```python
from build123d import *

# Parameters (mm, degrees)
F1_DEPTH = 50
F2_W     = 2.5
F2_H     = 40
F2_W_2   = 50
F2_W_3   = 9
F2_W_4   = 21.211368
F3_DEPTH = 5
F4_W     = 40
F4_H     = 40
F5_DEPTH = 350
F6_W     = 9
F6_H     = 40
F6_W_2   = 2.5
F7_DEPTH = 25


with BuildPart() as f1:
    # F0 (on Front) → F1 (new body)
    with BuildSketch(Plane.XZ):
        Polygon((97.859602, 45), (-152.140398, 45), (-152.140398, -5), (97.859602, -5), (97.859602, 0), align=None)
        Polygon((-147.140398, 40), (-145.640398, 40), (-125.92903, 0), (-147.140398, 0), align=None, mode=Mode.SUBTRACT)
        Polygon((-90.06627, 40), (-111.354901, 0), (-120.354901, 0), (-140.06627, 40), align=None, mode=Mode.SUBTRACT)
        Polygon((-55.690862, 0), (-105.690862, 0), (-84.402231, 40), (-75.402231, 40), align=None, mode=Mode.SUBTRACT)
        Polygon((-50.116734, 0), (-69.828102, 40), (-19.828102, 40), (-41.116734, 0), align=None, mode=Mode.SUBTRACT)
        Polygon((-14.164063, 40), (-5.164063, 40), (14.547306, 0), (-35.452694, 0), align=None, mode=Mode.SUBTRACT)
        Polygon((20.121434, 0), (0.410065, 40), (50.410065, 40), (29.121434, 0), align=None, mode=Mode.SUBTRACT)
        Polygon((65.074105, 40), (84.785473, 0), (34.785473, 0), (56.074105, 40), align=None, mode=Mode.SUBTRACT)
        Polygon((92.859602, 40), (92.859602, 0), (90.359602, 0), (70.648233, 40), align=None, mode=Mode.SUBTRACT)
    extrude(amount=F1_DEPTH)

    # F2 (on face) → F3 (cut)
    with BuildSketch(Plane(origin=(0, 0, -5), x_dir=(1, 0, 0), z_dir=(0, 0, -1))):
        with Locations((91.609602, 25)):
            Rectangle(F2_W, F2_H)
        with Locations((59.785473, 25)):
            Rectangle(F2_W_2, F2_H)
        with Locations((-10.452694, 25)):
            Rectangle(F2_W_2, F2_H)
        with Locations((24.621434, 25)):
            Rectangle(F2_W_3, F2_H)
        with Locations((-80.690862, 25)):
            Rectangle(F2_W_2, F2_H)
        with Locations((-45.616734, 25)):
            Rectangle(F2_W_3, F2_H)
        with Locations((-136.534714, 25)):
            Rectangle(F2_W_4, F2_H)
        with Locations((-115.854901, 25)):
            Rectangle(F2_W_3, F2_H)
    extrude(amount=-F3_DEPTH, mode=Mode.SUBTRACT)

    # F4 (on face) → F5 (cut)
    with BuildSketch(Plane.YZ.offset(97.859602)):
        with Locations((-25, 20)):
            Rectangle(F4_W, F4_H)
    extrude(amount=-F5_DEPTH, mode=Mode.SUBTRACT)

    # F6 (on face) → F7 (cut)
    with BuildSketch(Plane(origin=(0, 0, 40), x_dir=(1, 0, 0), z_dir=(0, 0, -1))):
        Polygon((-145.640398, 5), (-140.06627, 5), (-125.92903, 5), (-125.92903, 45), (-140.06627, 45), (-145.640398, 45), (-147.140398, 45), (-147.140398, 5), align=None)
        with Locations((-115.854901, 25)):
            Rectangle(F6_W, F6_H)
        Polygon((-5.164063, 5), (0.410065, 5), (14.547306, 5), (14.547306, 45), (0.410065, 45), (-5.164063, 45), (-14.164063, 45), (-19.828102, 45), (-35.452694, 45), (-35.452694, 5), (-19.828102, 5), (-14.164063, 5), align=None)
        Polygon((-75.402231, 5), (-69.828102, 5), (-55.690862, 5), (-55.690862, 45), (-69.828102, 45), (-75.402231, 45), (-84.402231, 45), (-90.06627, 45), (-105.690862, 45), (-105.690862, 5), (-90.06627, 5), (-84.402231, 5), align=None)
        with Locations((-45.616734, 25)):
            Rectangle(F6_W, F6_H)
        with Locations((24.621434, 25)):
            Rectangle(F6_W, F6_H)
        Polygon((65.074105, 5), (70.648233, 5), (84.785473, 5), (84.785473, 45), (70.648233, 45), (65.074105, 45), (56.074105, 45), (50.410065, 45), (34.785473, 45), (34.785473, 5), (50.410065, 5), (56.074105, 5), align=None)
        with Locations((91.609602, 25)):
            Rectangle(F6_W_2, F6_H)
    extrude(amount=-F7_DEPTH, mode=Mode.SUBTRACT)


solid = f1.part
```
Work out the finished part from the listing and answer in its coordinate system (mm). A direction names the side the tool comes from. Give positions to 0.01 mm unless a question says otherwise; leave off trailing zeros. Loops run counter-clockwise (first coordinate to the right, second up) from the corner with the lowest first, then second, coordinate; pieces in that order, holes last. Notation, with made-up numbers: M 85,-22.5 L 91,-22.5 A21 cw 91,1.5 Z; hole C 70,82.5 d4. An arc over 180 degrees is marked long. One line per item, written item: value. Start each with the question number.
1. Find section B-B (x = 38.5). Give the vertices of the cut face in (y, z).
2. Find the intervals of material crossed by probe 1 along Y at (x, z) = (42.5, 23.5); probe 2 along Z at (x, y) = (-36, -20); probe 3 along Z at (x, y) = (11, -3), in increasing order.
3. Find section A-A (x = -11.5). Give the vertices of the cut face in (y, z).
4. Each of these flat-tipped pins is pushed along its axis until it touches: P1, Ø8, axis at x = -132, z = 13, coming from the +Y side; P2, Ø1.5, axis at y = -37.5, z = 38.5, coming from the -X side. Where does it stop, or does it pass through?
5. Which of the six approach directions +Z, -Z, +X, -X, +Y, -Y give full straight-line access (tool end or side, diameter ignored) to faces 1 (the face through (-111.355, -25, 42)), 2 (the face through (-24.957, -47.465, 19.72)), 3 (the face through (-123, -25, 0))?
6. Find section C-C (y = -25.5). State how many separate pieces and enclosed holes the cut face has, and give its area (3 significant figures).
7. Determine the mould class of faces 4 (the face through (-120.355, -25, -3)), 5 (the face through (-80, -47, 0)) for opening direction Z: released by +Z, released by -Z, zero draft, split by the parting line, or undercut.
Reported:
1. outline: M -50,-5 L -45,-5 L -45,0 L -50,0 Z; M -50,6.98 L -45,6.98 L -45,17.62 L -50,17.62 Z; M -50,40 L -45,40 L -45,45 L -50,45 Z; M -5,-5 L 0,-5 L 0,0 L -5,0 Z; M -5,6.98 L 0,6.98 L 0,17.62 L -5,17.62 Z; M -5,40 L 0,40 L 0,45 L -5,45 Z
2. probe 1: y = -50 to -45, -5 to 0
2. probe 2: z = -5 to 0, 40 to 45
2. probe 3: z = -5 to 0, 7.2 to 18.51, 40 to 45
3. outline: M -50,-5 L -45,-5 L -45,0 L -50,0 Z; M -50,40 L -45,40 L -45,45 L -50,45 Z; M -5,-5 L 0,-5 L 0,0 L -5,0 Z; M -5,40 L 0,40 L 0,45 L -5,45 Z
4. P1: stops at y = 0
4. P2: passes through
5. face 1: +Z, -Z
5. face 2: +Y, -Y
5. face 3: +X, -X
6. separate pieces: 18
6. enclosed holes: 0
6. area: 493 mm²
7. face 4: zero draft
7. face 5: undercut
